Source: CAD feature listing. Evaluate the final solid. Frame: model axes, mm. Coordinates: 2 decimals unless noted, no trailing zeros. Order: outer loops, then holes, each group sorted by start corner. A loop starts at its lowest first (then second) coordinate and runs counter-clockwise, first axis right, second up. Notation, with made-up numbers: (40.25, 46.5) - (64.25, 46.5) arc R20 cw to (64.25, 71.5) - close; hole circle Ø4 at (56.5, -2). An arc over 180 degrees is marked (long way). One line per question, with ' | ' between items. Start each with the question number.
(1) Draft query along X for faces 1 (the flat face through (2, -2, -8.5)), 2 (the cylindrical face through (-0.867, 3.905, -0.116)), 3 (the cylindrical face through (2.003, 0.631, 0.116)). Return one class per face: +X half, -X half, draft (parallel to the pull), parting line (faces both ways), or undercut.
(2) Section C-C (z = 4). Return the cut outline in (x, y).
(3) Line query: line 1 along Y through (x, z) = (0, -1.75); line 2 along Y through (x, z) = (-0.5, 4.5); line 3 along X through (y, z) = (-0.75, -0.75). Output: solid intervals per line, ascending.
(4) Contact query for flat-ended pins moving along their axis: P1, Ø1, axis at y = -1, z = 4.5, coming from the -X side; P2, Ø1, axis at y = -1.5, z = 6, coming from the +X side; P3, Ø2, axis at y = 2.5, z = -1.5, coming from the +X side. Output: stop coordinate, or through.
(5) Section A-A (x = 0). Return the cut outline in (y, z).
Autodesk Inventor part; units mm, degrees
ref_plane "YZ Plane" through (0, 0, 0) normal (1, 0, 0) x (0, 1, 0)
ref_plane "XZ Plane" through (0, 0, 0) normal (0, 1, 0) x (-1, 0, 0)
ref_plane "XY Plane" through (0, 0, 0) normal (0, 0, 1) x (1, 0, 0)
sketch "スケッチ1" plane through (0, 0, 0) normal (0, 0, 1) x (1, 0, 0)
  circle A0 centre (0, 0) radius 2.1
  circle A1 centre (0, 0) radius 4
  dimension "d0" = 4.2
  dimension "d1" = 8
extrude "押し出し1" add sketch "スケッチ1" along normal mid plane 17
chamfer "面取り1" distance 0.2 angle 45 4 edges at (-2.1, 0, 8.5) (-4, 0, 8.5) (-4, 0, -8.5) (-2.1, 0, -8.5)
properties part number "CF-417E" material "鋼、炭素鋼"
Response values:
1) face 1: draft | face 2: parting line | face 3: undercut
2) outline: circle Ø8 at (0, 0); hole circle Ø4.2 at (0, 0)
3) line 1: y = -4 to -2.1, 2.1 to 4 | line 2: y = -3.97 to -2.04, 2.04 to 3.97 | line 3: x = -3.93 to -1.96, 1.96 to 3.93
4) P1: stops at x = -3.97 | P2: stops at x = 3.87 | P3: stops at x = 3.71
5) outline: (-4, -8.3) - (-3.8, -8.5) - (-2.3, -8.5) - (-2.1, -8.3) - (-2.1, 8.3) - (-2.3, 8.5) - (-3.8, 8.5) - (-4, 8.3) - close; (2.1, -8.3) - (2.3, -8.5) - (3.8, -8.5) - (4, -8.3) - (4, 8.3) - (3.8, 8.5) - (2.3, 8.5) - (2.1, 8.3) - close
